Verification items for the finished model (mm, model axes). A direction names the side the tool comes from. Round coordinates to 2 decimals unless told otherwise and drop trailing zeros. Loops run counter-clockwise (first coordinate to the right, second up) from the corner with the lowest first, then second, coordinate; pieces in that order, holes last. Notation, with made-up numbers: M -3.5,55.25 L 48.5,55.25 A21 cw 48.5,66.25 Z; hole C 53.25,36.25 d10. An arc over 180 degrees is marked long. Write item = value, one per line. Start each with the question number.
Autodesk Inventor part; units mm, degrees
ref_plane "YZ Plane" through (0, 0, 0) normal (1, 0, 0) x (0, 1, 0)
ref_plane "XZ Plane" through (0, 0, 0) normal (0, 1, 0) x (-1, 0, 0)
ref_plane "XY Plane" through (0, 0, 0) normal (0, 0, 1) x (1, 0, 0)
sketch "Sketch_2" plane through (0, 0, 0) normal (0, 0, 1) x (1, 0, 0)
  arc A0 (-20, 13.3) -> (-20, -13.3) centre (-20, 0) ccw
  line L0 (-20, -13.3) -> (290, -13.3)
  arc A1 (290, -13.3) -> (290, 13.3) centre (290, 0) ccw
  line L1 (290, 13.3) -> (-20, 13.3)
extrude "Extrusion1" add sketch "Sketch_2" along normal mid plane 10
sketch "Sketch_8" plane through (0, 0, 0) normal (0, 0, 1) x (1, 0, 0)
  line L0 (-1.5, 23.3) -> (-1.5, 13.3)
  line L1 (-1.5, 13.3) -> (1.5, 13.3)
  line L2 (1.5, 13.3) -> (1.5, 23.3)
  line L3 (1.5, 23.3) -> (-1.5, 23.3)
extrude "Extrusion2" add sketch "Sketch_8" along normal mid plane 9
sketch "_____3" plane through (0, 0, 0) normal (1, 0, 0) x (0, 0, -1)
  circle A0 centre (0, 18.8) radius 1.75
extrude "Extrusion3" cut sketch "_____3" along normal mid plane 6
sketch "_____2" plane through (0, 0, 0) normal (0, 0, 1) x (1, 0, 0)
  line L0 (33.5, 8.3) -> (36.5, 8.3)
  line L1 (36.5, 8.3) -> (36.5, 23.3)
  line L2 (36.5, 23.3) -> (33.5, 23.3)
  line L3 (33.5, 23.3) -> (33.5, 8.3)
extrude "Extrusion4" add sketch "_____2" along normal mid plane 9
sketch "Sketch5" plane through (33.5, 13.3, 4.5) normal (-1, 0, 0) x (0, 0, 1)
  point P0 (-4.5, 5.5)
hole "Hole1" at (33.5, 18.8, 0) direction (1, 0, 0) diameter 3.5 depth 3
sketch "Sketch_4" plane through (0, 0, 0) normal (0, 0, 1) x (1, 0, 0)
  arc A0 (-20, 12.3) -> (-20, -12.3) centre (-20, 0) ccw
  line L0 (-20, -12.3) -> (290, -12.3)
  arc A1 (290, -12.3) -> (290, 12.3) centre (290, 0) ccw
  line L1 (290, 12.3) -> (17.5, 12.3)
  line L2 (17.5, 12.3) -> (17.5, 11.1)
  line L3 (17.5, 11.1) -> (-7.5, 11.1)
  line L4 (-7.5, 11.1) -> (-7.5, 12.3)
  line L5 (-7.5, 12.3) -> (-20, 12.3)
extrude "Extrusion5" cut sketch "Sketch_4" along normal mid plane 10
sketch "Sketch_64" plane through (0, 0, 0) normal (0, 0, 1) x (1, 0, 0)
  line L0 (-9.3801, 11.1) -> (-9.3801, 10.1)
  line L1 (-9.3801, 10.1) -> (-5.6199, 10.1)
  line L2 (-5.6199, 10.1) -> (-5.6199, 11.1)
  arc A0 (-5.9958, 11.3632) -> (-5.6199, 11.1) centre (-5.6199, 11.5) ccw
  line L3 (-5.9958, 11.3632) -> (-6.241, 12.0368)
  arc A1 (-6.241, 12.0368) -> (-6.6168, 12.3) centre (-6.6168, 11.9) ccw
  line L4 (-6.6168, 12.3) -> (-7.125, 12.3)
  line L5 (-7.125, 12.3) -> (-7.125, 12.66)
  line L6 (-7.125, 12.66) -> (-7.875, 12.66)
  line L7 (-7.875, 12.66) -> (-7.875, 12.3)
  line L8 (-7.875, 12.3) -> (-8.3832, 12.3)
  arc A2 (-8.3832, 12.3) -> (-8.759, 12.0368) centre (-8.3832, 11.9) ccw
  line L9 (-8.759, 12.0368) -> (-9.0042, 11.3632)
  arc A3 (-9.3801, 11.1) -> (-9.0042, 11.3632) centre (-9.3801, 11.5) ccw
extrude "Extrusion6" cut sketch "Sketch_64" along normal mid plane 10
pattern_linear "Rectangular Pattern1" count 6 spacing 5 along (1, 0, 0) of "Extrusion6"
properties part number "ATBT-700T5100-B-P35_info-1-16-16"
1. Thickness scan on line 1 (Y direction, x = 30.5, z = 3); line 2 (X direction, y = 20, z = -4); line 3 (Z direction, x = -0.55, y = 18.8). Record the ranges inside material, lowest first.
2. Section check B-B, the plane x = 148. Enter the section's corners in (y, z).
3. Gauge pin test, flat ends, axial feed: P1, Ø4, axis at y = 12.5, z = 2, coming from the +X side; P2, Ø6, axis at y = -6, z = 2.5, coming from the +X side; P3, Ø2, axis at y = -3, z = 1, coming from the -X side. Record the tip position at first contact, or that the pin passes through.
4. Mould release check, pull along X, two halves, no side actions. Record for faces 6 (the flat face through (133, -12.3, 0)), 7 (the flat face through (36.5, 17, 1)), 8 (the flat face through (133, -13.3, 0)): pulls with the +X half, pulls with the -X half, needs draft (parallel to the pull), parting line crosses it, or undercut.
5. Section check A-A, the plane y = 0. Enter the section's corners in (x, z).
6. Tool access check on faces 1 (the cylindrical face through (-32.297, -0.27, -0.07)), 2 (the flat face through (-1.5, 17, -1)), 3 (the flat face through (33.5, 17, -1)), 4 (the cylindrical face through (-33.297, -0.292, -0.07)), 5 (the cylindrical face through (303.297, 0.292, -0.07)). Record the directions out of +Z, -Z, +X, -X, +Y, -Y that give a thin tool (end or side, any length) a straight path to the whole face; none if there is none.
Computed values:
q1.line_1 = -13.3 to -12.3, 12.3 to 13.3
q1.line_2 = -1.5 to 1.5, 33.5 to 36.5
q1.line_3 = -4.5 to -1.75, 1.75 to 4.5
q2.outline = M -13.3,-5 L -12.3,-5 L -12.3,5 L -13.3,5 Z; M 12.3,-5 L 13.3,-5 L 13.3,5 L 12.3,5 Z
q3.P1 = 298.16
q3.P2 = 302.96
q3.P3 = -33.15
q4.face_6 = undercut
q4.face_7 = pulls with the +X half
q4.face_8 = needs draft
q5.outline = M -33.3,-5 L -32.3,-5 L -32.3,5 L -33.3,5 Z; M 302.3,-5 L 303.3,-5 L 303.3,5 L 302.3,5 Z
q6.face_1 = +Z, -Z
q6.face_2 = +Z, -Z, -X, +Y
q6.face_3 = +Z, -Z, +Y
q6.face_4 = +Z, -Z, -X
q6.face_5 = +Z, -Z, +X
